Read the model definition and answer for the solid it produces. Units are mm, in the model's axes. Face numbers are marked on the shaded views. Coordinates: 2 decimals unless noted, no trailing zeros. Order: outer loops, then holes, each group sorted by start corner. A loop starts at its lowest first (then second) coordinate and runs counter-clockwise, first axis right, second up. Notation, with made-up numbers: (-7, 25.25) - (46, 25.25) arc R20 ccw to (46, 45.25) - close; hole circle Ø9 at (80, 59). An arc over 180 degrees is marked (long way). Use one line per item in the form item = value.
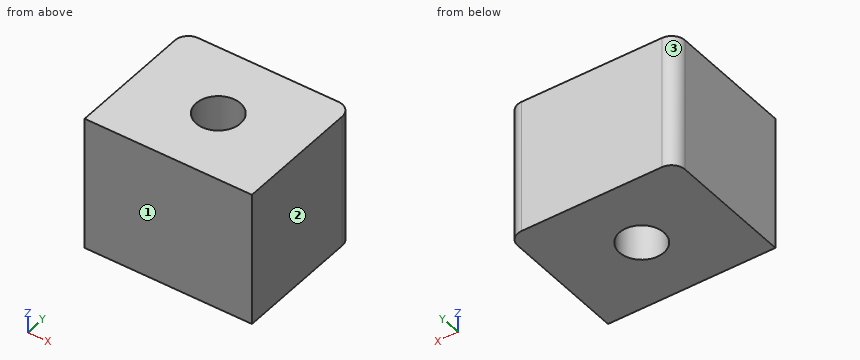
```python
from build123d import *

# Parameters (mm, degrees)
F0_W          = 63.1906017661
F0_H          = 52.1872714162
F0_R          = 8.3960945755
F1_DEPTH      = 25.4
F1_DEPTH_BACK = 25.4
F2_R          = 5.08


# Not quite as in the source:
# - the program builds the solid bodies; features that only make, move or delete a surface that nothing else refers to are left out


with BuildPart() as f1:
    # F0 (on Top) → F1 (new body, two sides)
    with BuildSketch(Plane.XY) as f1_sk:
        Rectangle(F0_W, F0_H)
        Circle(F0_R, mode=Mode.SUBTRACT)
    extrude(amount=F1_DEPTH)
    extrude(f1_sk.sketch, amount=-F1_DEPTH_BACK)

    # F2
    f2_edges = [f1.edges().sort_by_distance(p)[0] for p in [
        (-31.595301, 26.093636, 0),
        (31.595301, 26.093636, 0),
    ]]
    fillet(f2_edges, radius=F2_R)


solid = f1.part
```
(1) Section A-A, the plane x = 0 is taken. Write down the section's boundary in (y, z).
Answer list:
outline = (-26.09, -25.4) - (-8.4, -25.4) - (-8.4, 25.4) - (-26.09, 25.4) - close; (8.4, -25.4) - (26.09, -25.4) - (26.09, 25.4) - (8.4, 25.4) - close
(2) Section C-C, the plane y = 0 is taken. Write down the section's boundary in (x, z).
Answer list:
outline = (-31.6, -25.4) - (-8.4, -25.4) - (-8.4, 25.4) - (-31.6, 25.4) - close; (8.4, -25.4) - (31.6, -25.4) - (31.6, 25.4) - (8.4, 25.4) - close
(3) Straight lines are drawn through the part: L1, parallel to X at y = -0.5, z = 5.5; L2, parallel to Y at x = 0, z = 8; L3, parallel to Y at x = 3.5, z = 5.5. For each, find the intervals that lie inside material, in ascending order.
Answer list:
L1 = -31.6 to -8.38, 8.38 to 31.6
L2 = -26.09 to -8.4, 8.4 to 26.09
L3 = -26.09 to -7.63, 7.63 to 26.09
(4) Section B-B, the plane z = -4 is taken. Write down the section's boundary in (x, y), then the cut area to 3 significant figures.
Answer list:
outline = (-31.6, -26.09) - (31.6, -26.09) - (31.6, 21.01) arc R5.08 ccw to (26.52, 26.09) - (-26.52, 26.09) arc R5.08 ccw to (-31.6, 21.01) - close; hole circle Ø16.79 at (0, 0)
area = 3,070 mm2
(5) The mould has two halves that part along Y. Classify the marked faces 1, 2 and 3: +Y half, -Y half, draft (parallel to the pull), parting line (faces both ways), or undercut.
Answer list:
face_1 = -Y half
face_2 = draft
face_3 = +Y half
